from build123d import *

# Parameters (mm, degrees)
F1_DEPTH      = 25.4
F3_DEPTH      = 19.05
F4_R          = 5.08
F5_R          = 3.175
F6_DEPTH      = 87.203302
F6_DEPTH_BACK = 87.203302
F7_DEPTH      = 38.1
F8_R          = 2.54
F9_DEPTH      = 125.303302


with BuildPart() as f1:
    # F0 (on Top) → F1 (new body)
    with BuildSketch(Plane.XY):
        Polygon((-43.994091, -76.2), (43.994091, -76.2), (87.988181, 0), (43.994091, 76.2), (-43.994091, 76.2), (-87.988181, 0), align=None)
    extrude(amount=F1_DEPTH)

    # F2 (on face) → F3 (cut)
    with BuildSketch(Plane.XY.offset(25.4)):
        Polygon((-7.332348, -12.7), (7.332348, -12.7), (14.664697, 0), (7.332348, 12.7), (-7.332348, 12.7), (-14.664697, 0), align=None)
        Polygon((-7.332348, 38.1), (7.332348, 38.1), (14.664697, 50.8), (7.332348, 63.5), (-7.332348, 63.5), (-14.664697, 50.8), align=None)
        Polygon((-29.329394, 25.4), (-36.661742, 38.1), (-51.326439, 38.1), (-58.658787, 25.4), (-51.326439, 12.7), (-36.661742, 12.7), align=None)
        Polygon((-36.661742, -12.7), (-51.326439, -12.7), (-58.658787, -25.4), (-51.326439, -38.1), (-36.661742, -38.1), (-29.329394, -25.4), align=None)
        Polygon((-7.332348, -38.1), (-14.664697, -50.8), (-7.332348, -63.5), (7.332348, -63.5), (14.664697, -50.8), (7.332348, -38.1), align=None)
        Polygon((29.329394, -25.4), (36.661742, -38.1), (51.326439, -38.1), (58.658787, -25.4), (51.326439, -12.7), (36.661742, -12.7), align=None)
        Polygon((36.661742, 12.7), (51.326439, 12.7), (58.658787, 25.4), (51.326439, 38.1), (36.661742, 38.1), (29.329394, 25.4), align=None)
    extrude(amount=-F3_DEPTH, mode=Mode.SUBTRACT)

    # F4
    f4_edges = [f1.edges().sort_by_distance(p)[0] for p in [
        (0, -76.2, 0),
        (65.991136, -38.1, 0),
        (65.991136, 38.1, 0),
        (0, 76.2, 0),
        (-65.991136, 38.1, 0),
        (-65.991136, -38.1, 0),
        (43.994091, -76.2, 12.7),
        (87.988181, 0, 12.7),
        (-43.994091, -76.2, 12.7),
        (-43.994091, 76.2, 12.7),
        (43.994091, 76.2, 12.7),
        (-87.988181, 0, 12.7),
    ]]
    fillet(f4_edges, radius=F4_R)

    # F5 (on Right) → F6 (cut, two sides)
    with BuildSketch(Plane.YZ) as f6_sk:
        with Locations((76.11011, 25.39102)):
            Circle(F5_R)
    extrude(amount=F6_DEPTH, mode=Mode.SUBTRACT)
    extrude(f6_sk.sketch, amount=-F6_DEPTH_BACK, mode=Mode.SUBTRACT)

    # F5 (on Right) → F7 (join)
    with BuildSketch(Plane.YZ):
        with Locations((76.11011, 25.39102)):
            Circle(F5_R)
    extrude(amount=F7_DEPTH)

    # F8 (on face) → F9 (cut, through all)
    with BuildSketch(Plane.YZ.offset(38.1)):
        with Locations((76.11011, 25.39102)):
            Circle(F8_R)
    extrude(amount=-F9_DEPTH, mode=Mode.SUBTRACT)


solid = f1.part
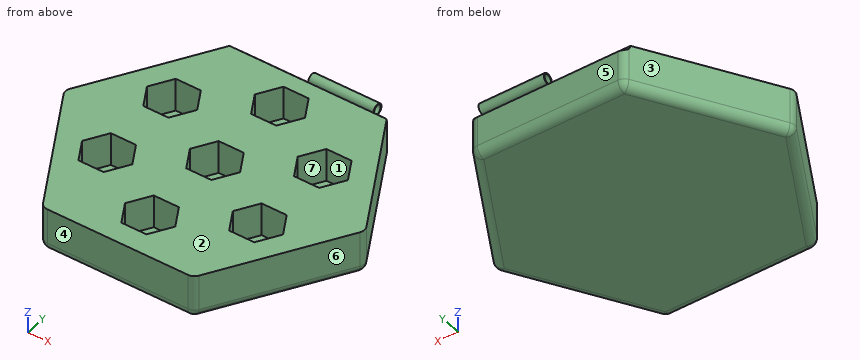
For this review, take the finished solid that the model builds, in its own axes (mm). Face numbers are marked on the shaded views. A direction names the side the tool comes from. Round coordinates to 2 decimals unless told otherwise and drop trailing zeros. Loops run counter-clockwise (first coordinate to the right, second up) from the corner with the lowest first, then second, coordinate; pieces in that order, holes last. Notation, with made-up numbers: (-32, 15) - (-6, 15) arc R16 ccw to (-6, 29) - close; hole circle Ø1 at (53.5, -38). An arc over 180 degrees is marked (long way). Use one line per item in the form item = value.
1) Tool access review of the marked faces 5, 6 and 7: name each direction out of +Z, -Z, +X, -X, +Y, -Y from which nothing blocks a thin tool from reaching the whole face with its end or side.
Solutions:
face_5 = -Z, +X, -X, +Y
face_6 = +Z, -Z, +X, -Y
face_7 = +Z
2) Wall thickness on probe 1 along Y at (x, z) = (5.5, 13); probe 2 along Y at (x, z) = (32, 22.75); probe 3 along X at (y, z) = (-22.5, 17.5): over which ranges is each line inside the solid? List them lowest first.
Solutions:
probe_1 = -76.2 to -63.5, -38.1 to -12.7, 12.7 to 38.1, 63.5 to 76.2
probe_2 = -76.2 to -30.03, -20.77 to 20.77, 30.03 to 77.87
probe_3 = -75 to -56.98, -31 to 31, 56.98 to 75
3) Mouldability with a two-part tool opening along Y and no side actions: class the marked faces 1, 2, 3 and 4 as pulls with the +Y half, pulls with the -Y half, needs draft (parallel to the pull), parting line crosses it, or undercut.
Solutions:
face_1 = undercut
face_2 = needs draft
face_3 = pulls with the +Y half
face_4 = pulls with the -Y half
4) Clearance check with flat-ended pins moving along their axes: P1, Ø5, axis at y = 22.5, z = 3.5, coming from the -X side; P2, Ø3, axis at y = 75, z = 24.5, coming from the -X side; P3, Ø16, axis at x = -2.5, z = 17.5, coming from the +Y side; P4, Ø1.5, axis at x = -53, y = -7.5, coming from the -Z side. State where each tip first meets the part, or that it passes through.
Solutions:
P1 = -76.3
P2 = 0
P3 = 79.27
P4 = 0
5) We need section B-B on z = 20. State how many separate pieces and enclosed holes the cut face has, then the cut area to 3 significant figures.
Solutions:
separate_pieces = 1
enclosed_holes = 7
area = 16,200 mm2
6) We need section A-A on x = 32. Write out the cut boundary in (y, z) (3 decimals).
Solutions:
outline = (-76.2, 5.08) arc R5.08 ccw to (-71.12, 0) - (71.12, 0) arc R5.08 ccw to (76.2, 5.08) - (76.2, 22.217) arc R3.175 ccw (long way) to (72.935, 25.4) - (30.026, 25.4) - (30.026, 6.35) - (20.774, 6.35) - (20.774, 25.4) - (-20.774, 25.4) - (-20.774, 6.35) - (-30.026, 6.35) - (-30.026, 25.4) - (-76.2, 25.4) - close; hole circle Ø5.08 at (76.11, 25.391)
